Part model, mm, in its own coordinate system. A direction names the side the tool comes from. Give positions to 0.01 mm unless a question says otherwise; leave off trailing zeros. Order: outer loops, then holes, each group sorted by start corner. A loop starts at its lowest first (then second) coordinate and runs counter-clockwise, first axis right, second up. Notation, with made-up numbers: (-5.75, 85) -> (49.25, 85) arc R11 cw to (49.25, 90) -> close; hole circle Ø8 at (20, 61). An arc over 180 degrees is marked (long way). Write item = value, one per line. Start each with the question number.
Item 1: Band-saw the part on A-A on x = -11. Write the cut outline in (y, z), plus the area to 3 significant figures.
Item 2: Drill centre lines: line 1 along Y through (x, z) = (3.5, -9); line 2 along Z through (x, y) = (2, 21.5); line 3 along Y through (x, z) = (-16.5, -18). Where is each one in solid material? Low to high.
Item 3: Tool access for faces 1 (the face through (25.4, 13, -23)), 2 (the face through (0, 27, -22.23)): list every direction of +Z, -Z, +X, -X, +Y, -Y with a clear straight run to the whole face (end or side of a thin tool).
Item 4: Flat gauge pins, fed straight in: P1, Ø1, axis at x = -8.5, z = -21, coming from the +Y side; P2, Ø5, axis at x = -18.5, z = -16, coming from the +Y side; P3, Ø5, axis at x = 17, y = 26.5, coming from the +Z side. Where does each tip first touch, or does it go through?
Item 5: Band-saw the part on B-B on y = 44. Write the cut outline in (x, z).
Item 6: Band-saw the part on C-C on z = -6. Write the cut outline in (x, y), plus the area to 3 significant figures.
```python
from build123d import *

# Parameters (mm, degrees)
BOSS_EXTRUDE1_DEPTH = 25.4
FILLET1_R           = 6.25


with BuildPart() as part:
    # Sketch1 → Boss-Extrude1 (new body, symmetric)
    with BuildSketch(Plane(origin=(0, 0, 0), x_dir=(0, 0, -1), z_dir=(1, 0, 0))):
        Polygon((0, 0), (22.23, 0), (22.23, 47.63), (25.4, 47.63), (25.4, -3.17), (0, -3.17), align=None)
    extrude(amount=BOSS_EXTRUDE1_DEPTH, both=True)

    # Fillet1
    fillet1_edges = [part.edges().sort_by_distance(p)[0] for p in [
        (0, 0, -22.23),
    ]]
    fillet(fillet1_edges, radius=FILLET1_R)


solid = part.part
```
Values found:
q1.outline = (-3.17, -25.4) -> (47.63, -25.4) -> (47.63, -22.23) -> (6.25, -22.23) arc R6.25 cw to (0, -15.98) -> (0, 0) -> (-3.17, 0) -> close
q1.area = 240 mm^2
q2.line_1 = -3.17 to 0
q2.line_2 = -25.4 to -22.23
q2.line_3 = -3.17 to 0.34
q3.face_1 = +Z, -Z, +X, +Y, -Y
q3.face_2 = +Z, +X, -X, +Y
q4.P1 = 3.32
q4.P2 = 0.53
q4.P3 = -22.23
q5.outline = (-25.4, -25.4) -> (25.4, -25.4) -> (25.4, -22.23) -> (-25.4, -22.23) -> close
q6.outline = (-25.4, -3.17) -> (25.4, -3.17) -> (25.4, 0) -> (-25.4, 0) -> close
q6.area = 161 mm^2
